Verification items for the finished model (mm, model axes). Round coordinates to 2 decimals unless told otherwise and drop trailing zeros. Order: outer loops, then holes, each group sorted by start corner. A loop starts at its lowest first (then second) coordinate and runs counter-clockwise, first axis right, second up. Notation, with made-up numbers: (2.25, 81) -> (51.25, 81) arc R22 cw to (51.25, 118) -> close; hole circle Ø5 at (87, 62.5). An arc over 180 degrees is marked (long way). Write item = value, one per line. Start each with the question number.
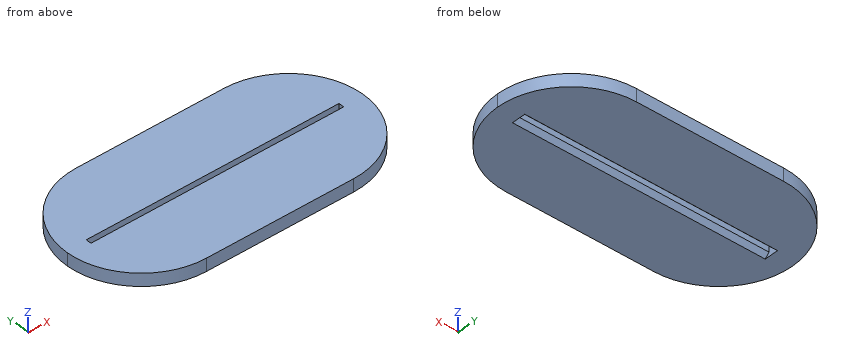
from build123d import *

# Parameters (mm, degrees)
F0_W     = 70
F0_H     = 35
F0_W_2   = 60
F0_H_2   = 1.3
F1_DEPTH = 3
F2_R     = 17.49999
F3_SIZE  = 1


# Not quite as in the source:
# - a fillet or chamfer is up to 0.001 mm smaller than in the source, because OpenCascade refuses the exact size


with BuildPart() as f1:
    # F0 (on Top) → F1 (new body)
    with BuildSketch(Plane.XY):
        with Locations((35, 17.5)):
            Rectangle(F0_W, F0_H)
        with Locations((35, 17.5)):
            Rectangle(F0_W_2, F0_H_2, mode=Mode.SUBTRACT)
    extrude(amount=F1_DEPTH)

    # F2 (radius 17.5 in the source; OpenCascade refuses exactly that, so slightly less here)
    f2_edges = [f1.edges().sort_by_distance(p)[0] for p in [
        (70, 0, 1.5),
        (70, 35, 1.5),
        (0, 35, 1.5),
        (0, 0, 1.5),
    ]]
    fillet(f2_edges, radius=F2_R)

    # F3
    f3_edges = [f1.edges().sort_by_distance(p)[0] for p in [
        (35, 16.85, 0),
        (35, 18.15, 0),
    ]]
    chamfer(f3_edges, length=F3_SIZE)


solid = f1.part
(1) Scan lines: line 1 along Y through (x, z) = (34.5, 1.1); line 2 along X through (y, z) = (17, 1.6); line 3 along Y through (x, z) = (49, 0.5). Record each from-to range of solid material in increasing order. Write a range as from..to.
(2) Depth check by flat-ended pin: pin 1 (1.5 mm diameter, centred on y = 18, z = 2, fed in from +X). Enter the tip coordinate at first touch or a pass-through.
(3) Cross-section at A-A (x = 19.5). Enter the section's corners in (y, z), and give its area (3 significant figures).
(4) Cross-section at C-C (y = 7). Enter the section's corners in (x, z).
(5) Cross-section at D-D (x = 58.5). Enter the section's corners in (y, z), and give its area (3 significant figures).
Outcome:
q1.line_1 = 0..16.85, 18.15..35
q1.line_2 = 0.01..5, 65..69.99
q1.line_3 = 0..16.35, 18.65..35
q2.pin_1 = 70
q3.outline = (0, 0) -> (15.85, 0) -> (16.85, 1) -> (16.85, 3) -> (0, 3) -> close; (18.15, 1) -> (19.15, 0) -> (35, 0) -> (35, 3) -> (18.15, 3) -> close
q3.area = 100 mm^2
q4.outline = (3.5, 0) -> (66.5, 0) -> (66.5, 3) -> (3.5, 3) -> close
q5.outline = (1.06, 0) -> (15.85, 0) -> (16.85, 1) -> (16.85, 3) -> (1.06, 3) -> close; (18.15, 1) -> (19.15, 0) -> (33.94, 0) -> (33.94, 3) -> (18.15, 3) -> close
q5.area = 93.7 mm^2
